Design review of the part shown in the three views and the two pictorial views. Dimensions are in mm from the part's minimum x, y and z. Round coordinates to 2 decimals unless told otherwise and drop trailing zeros. Loops run counter-clockwise (first coordinate to the right, second up) from the corner with the lowest first, then second, coordinate; pieces in that order, holes last.
1. Consider section A-A on x = 63.5. State the section outline as (y, z) points.
2. Clearance check with flat-ended pins moving along their axes: pin 1 Ø10 at (x, y) = (17, 56) entering from +Z; pin 2 Ø2 at (x, y) = (14.5, 43.5) entering from +Z; pin 3 Ø0.8 at (y, z) = (29.5, 1) entering from +X. State where each tip first meets the part, or that it passes through.
3. To check wall thickness, follow line 1 along Y through (x, z) = (40.5, 0.55); line 2 along X through (y, z) = (62.5, 0.6). State the ranges of each line that lie inside material, in increasing order.
4. Consider section B-B on y = 6.35. State the section outline as (x, z) points.
5. Consider section D-D on z = 1. State how many separate pieces and enclosed holes the cut face has, then the cut area to 3 significant figures.
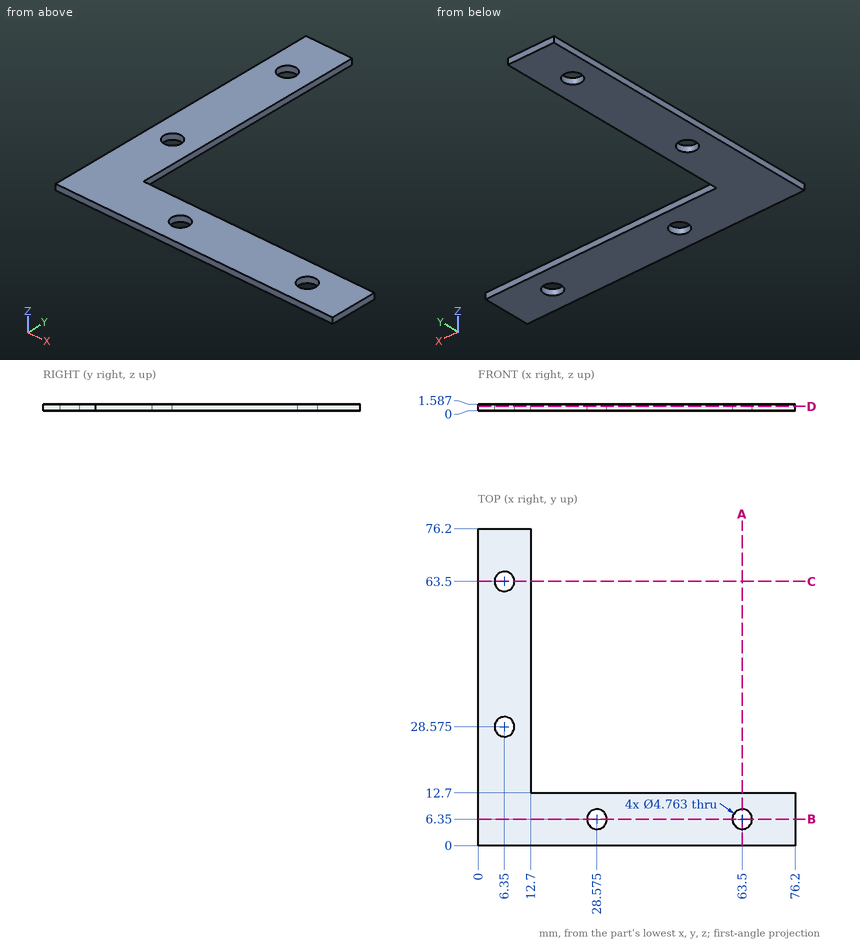
Resolved:
1. outline: (0, 0) - (3.97, 0) - (3.97, 1.59) - (0, 1.59) - close; (8.73, 0) - (12.7, 0) - (12.7, 1.59) - (8.73, 1.59) - close
2. pin 1: stops at z = 1.59
2. pin 2: passes through
2. pin 3: stops at x = 12.7
3. line 1: y = 0 to 12.7
3. line 2: x = 0 to 4.19, 8.51 to 12.7
4. outline: (0, 0) - (26.19, 0) - (26.19, 1.59) - (0, 1.59) - close; (30.96, 0) - (61.12, 0) - (61.12, 1.59) - (30.96, 1.59) - close; (65.88, 0) - (76.2, 0) - (76.2, 1.59) - (65.88, 1.59) - close
5. separate pieces: 1
5. enclosed holes: 4
5. area: 1,700 mm2
